Here's the drawing with two shaded views (mm, measured from the low corner). I have some questions. A direction names the side the tool comes from. Give positions to 0.01 mm unless a question says otherwise; leave off trailing zeros. Loops run counter-clockwise (first coordinate to the right, second up) from the corner with the lowest first, then second, coordinate; pieces in that order, holes last. Notation, with made-up numbers: M 13.25,76.5 L 18.25,76.5 A30 cw 18.25,103.5 Z; hole C -11,43 d9. An arc over 180 degrees is marked long. Use CSV: the item, a comma, the result in double quotes.
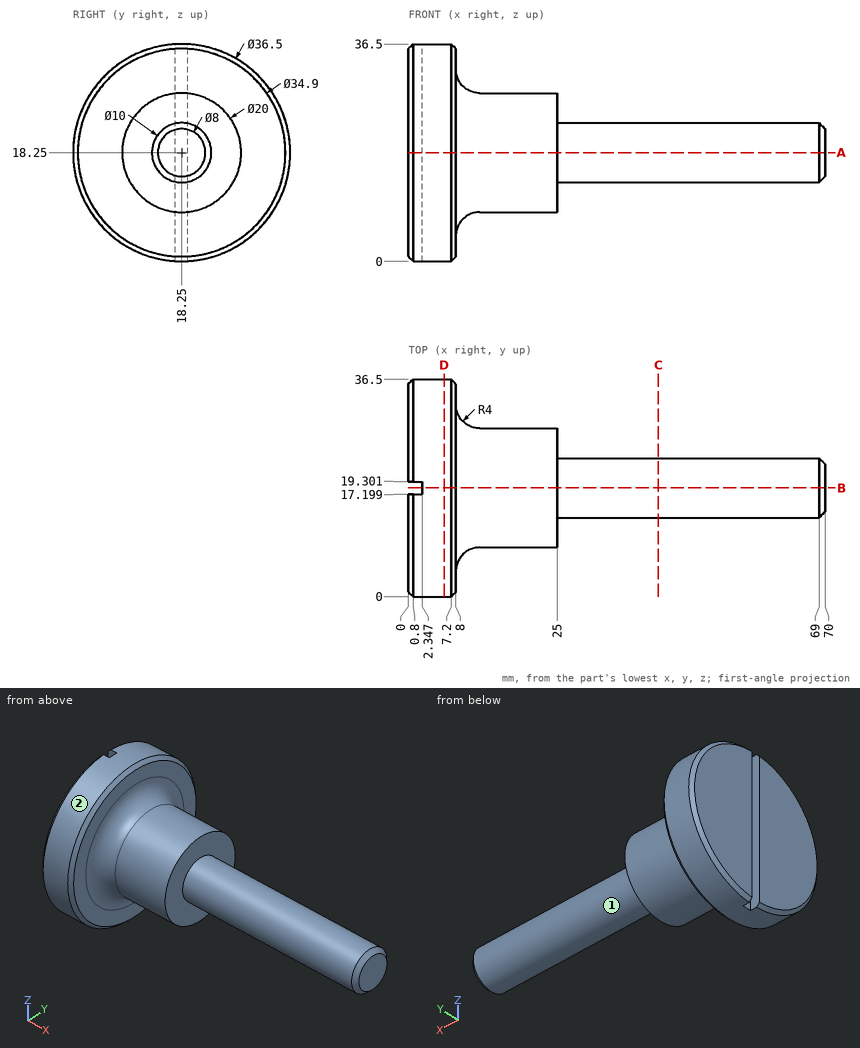
1. I want a section at A-A, the plane z = 18.25. List the corners of the cut face in (x, y) for me, then the cut area to 3 significant figures.
Outcome:
outline,"M 0,0.8 L 0.8,0 L 7.2,0 L 8,0.8 L 8,4.25 A4 cw 12,8.25 L 25,8.25 L 25,13.25 L 69,13.25 L 70,14.25 L 70,22.25 L 69,23.25 L 25,23.25 L 25,28.25 L 12,28.25 A4 cw 8,32.25 L 8,35.7 L 7.2,36.5 L 0.8,36.5 L 0,35.7 L 0,19.3 L 2.35,19.3 L 2.35,17.2 L 0,17.2 Z"
area,"1,080 mm2"
2. I want a section at B-B, the plane y = 18.25. List the corners of the cut face in (x, z) for me.
Outcome:
outline,"M 2.35,0 L 7.2,0 L 8,0.8 L 8,4.25 A4 cw 12,8.25 L 25,8.25 L 25,13.25 L 69,13.25 L 70,14.25 L 70,22.25 L 69,23.25 L 25,23.25 L 25,28.25 L 12,28.25 A4 cw 8,32.25 L 8,35.7 L 7.2,36.5 L 2.35,36.5 Z"
3. Which directions (+Z, -Z, +X, -X, +Y, -Y) give clear straight access to the entire face, cutting with the end or side of a thin tool? Please do the marked faces 1 and 2.
Outcome:
face 1,"+X"
face 2,"+X, -X"
4. Please list where these lines run through material, in increasing order: line 1 (X direction, y = 23, z = 24.5); line 2 (X direction, y = 12, z = 3); line 3 (Z direction, x = 26, y = 21) (1 decimal).
Outcome:
line 1,"0 to 25"
line 2,"0 to 8"
line 3,"14.1 to 22.4"
5. I want a section at D-D, the plane x = 6. List the corners of the cut face in (y, z) for me, then the cut area to 3 significant figures.
Outcome:
outline,"C 18.25,18.25 d36.5"
area,"1,050 mm2"
6. I want a section at C-C, the plane x = 42. List the corners of the cut face in (y, z) for me.
Outcome:
outline,"C 18.25,18.25 d10"
7. I'm going to push flat-ended pins straight in: pin 1 Ø6 at (y, z) = (23, 22.5) entering from +X; pin 2 Ø1 at (x, z) = (49.5, 21.5) entering from +Y (1 decimal); pin 3 Ø1.2 at (x, z) = (1.5, 24.5) entering from +Y; pin 4 Ø4 at (x, z) = (58.5, 16) entering from +Y. Where does each tip first touch, or does it pass through?
Outcome:
pin 1,"x = 70"
pin 2,"y = 22.4"
pin 3,"y = 35.6"
pin 4,"y = 23.24"
